Job drawing, mm, ordinate dimensions from the low corner. One solid piece. A direction names the side the tool comes from. Give positions to 0.01 mm unless a question says otherwise; leave off trailing zeros. Order: outer loops, then holes, each group sorted by start corner. A loop starts at its lowest first (then second) coordinate and runs counter-clockwise, first axis right, second up. Notation, with made-up numbers: (1, 80) - (30, 80) arc R15 cw to (30, 104) - close; hole circle Ø2 at (65.25, 86.25). An arc over 180 degrees is marked (long way). Write each question's results on one line, items separated by ' | '. Start each with the question number.
1) Two-plate mould, pull along Y, no slides. Class the marked faces 1, 2, 3 and 4: +Y half, -Y half, draft (parallel to the pull), parting line (faces both ways), or undercut.
2) Cut at A-A on x = 20. List the corners of the cut face in (y, z), plus the area to 3 significant figures.
3) Tool access for the marked faces 5 and 6: list every direction of +Z, -Z, +X, -X, +Y, -Y with a clear straight run to the whole face (end or side of a thin tool).
4) Cut at C-C on z = 105.5. List the corners of the cut face in (x, y), plus the area to 3 significant figures.
5) Drill centre lines: line 1 along X through (y, z) = (33.5, 116); line 2 along Y through (x, z) = (36, 66). Where is each one in solid material? Low to high. Write a range as from..to.
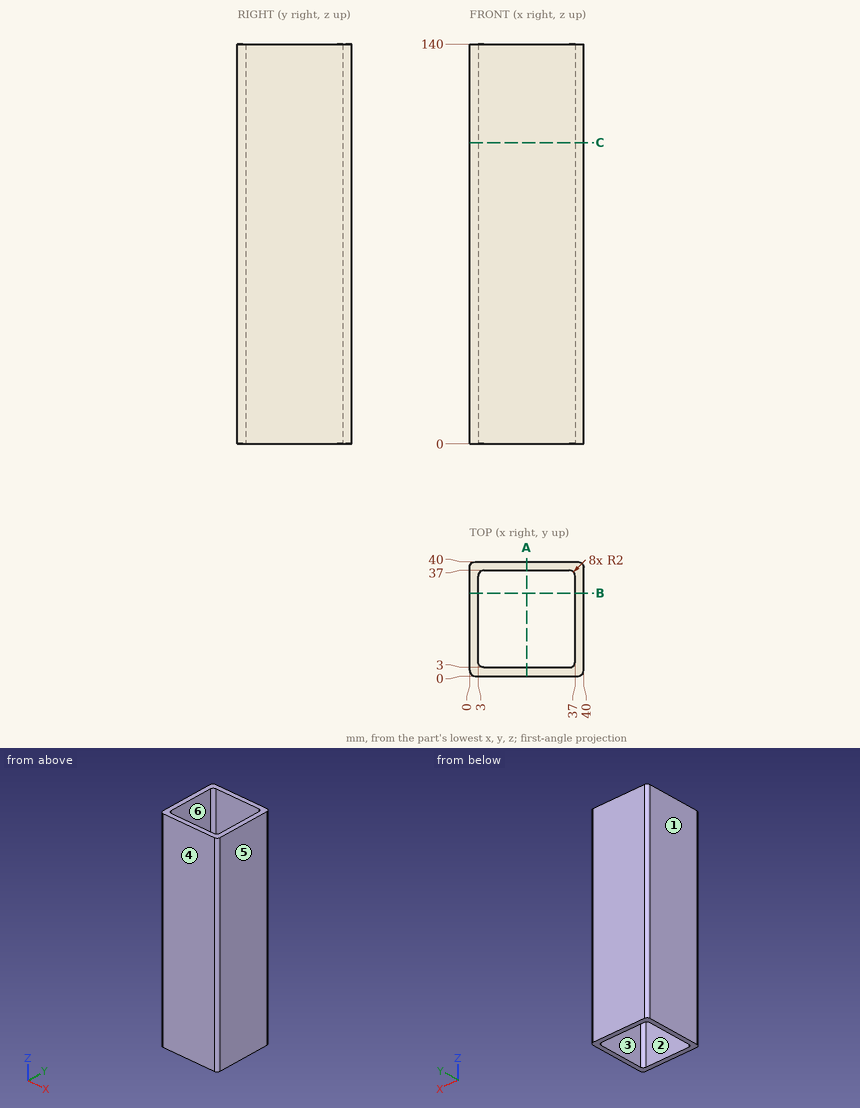
Results:
1) face 1: draft | face 2: undercut | face 3: undercut | face 4: -Y half
2) outline: (0, 0) - (3, 0) - (3, 140) - (0, 140) - close; (37, 0) - (40, 0) - (40, 140) - (37, 140) - close | area: 840 mm^2
3) face 5: +Z, -Z, +X, +Y, -Y | face 6: +Z, -Z
4) outline: (0, 2) arc R2 ccw to (2, 0) - (38, 0) arc R2 ccw to (40, 2) - (40, 38) arc R2 ccw to (38, 40) - (2, 40) arc R2 ccw to (0, 38) - close; hole (3, 5) arc R2 ccw to (5, 3) - (35, 3) arc R2 ccw to (37, 5) - (37, 35) arc R2 ccw to (35, 37) - (5, 37) arc R2 ccw to (3, 35) - close | area: 444 mm^2
5) line 1: 0..3, 37..40 | line 2: 0..3.27, 36.73..40
